CAD build for the part. Positions are in the model's coordinates, mm. Face numbers are marked on the shaded views. A direction names the side the tool comes from. Round coordinates to 2 decimals unless told otherwise and drop trailing zeros. Order: outer loops, then holes, each group sorted by start corner. A loop starts at its lowest first (then second) coordinate and runs counter-clockwise, first axis right, second up. Notation, with made-up numbers: M 33.5,-13 L 64.5,-13 A24 cw 64.5,1 Z; hole C 28.25,55 d4. An arc over 180 degrees is marked long. Answer as a JSON object with one key per item and string values.
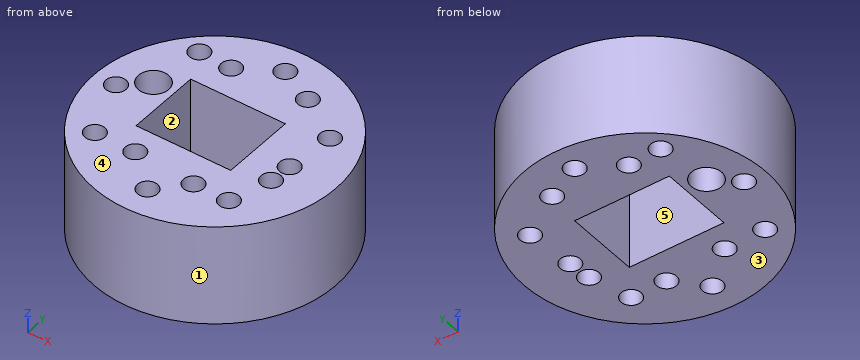
```python
from build123d import *

# Parameters (mm, degrees)
F0_R      = 30
F1_DEPTH  = 25
F2_W      = 23.500042
F2_H      = 18.234876
F3_DEPTH  = 15
F4_DEPTH  = 25
F5_R      = 2.5
F5_R_2    = 3.773073
F6_DEPTH  = 25
F7_R      = 2.5
F8_DEPTH  = 25
F9_R      = 2.5
F10_DEPTH = 25
F11_R     = 2.5
F12_DEPTH = 25


with BuildPart() as f1:
    # F0 (on Top) → F1 (new body)
    with BuildSketch(Plane.XY):
        Circle(F0_R)
    extrude(amount=F1_DEPTH)

    # F2 (on face) → F3 (join)
    with BuildSketch(Plane.XY.offset(25)):
        with Locations((-1.940479, 1.186641)):
            Rectangle(F2_W, F2_H)
    extrude(amount=-F3_DEPTH)

    # F2 (on face) → F4 (cut)
    with BuildSketch(Plane.XY.offset(25)):
        with Locations((-1.940479, 1.186641)):
            Rectangle(F2_W, F2_H)
    extrude(amount=-F4_DEPTH, mode=Mode.SUBTRACT)

    # F5 (on face) → F6 (cut)
    with BuildSketch(Plane.XY.offset(25)):
        with Locations((0, -22.529673)):
            Circle(F5_R)
        with Locations((18.548569, 0)):
            Circle(F5_R)
        with Locations((8.835036, 19.124642)):
            Circle(F5_R)
        with Locations((-19.018844, -14.531934)):
            Circle(F5_R)
        with Locations((-19.018844, 5.049379)):
            Circle(F5_R_2)
    extrude(amount=-F6_DEPTH, mode=Mode.SUBTRACT)

    # F7 (on face) → F8 (cut)
    with BuildSketch(Plane.XY.offset(25)):
        with Locations((-9.274186, 17.875323)):
            Circle(F7_R)
        with Locations((0, 23.479404)):
            Circle(F7_R)
        with Locations((15.148347, -15.728295)):
            Circle(F7_R)
    extrude(amount=-F8_DEPTH, mode=Mode.SUBTRACT)

    # F9 (on face) → F10 (cut)
    with BuildSketch(Plane.XY.offset(25)):
        with Locations((-8.938282, -14.577557)):
            Circle(F9_R)
        with Locations((19.652629, 11.967526)):
            Circle(F9_R)
        with Locations((6.387524, -15.767302)):
            Circle(F9_R)
        with Locations((-24.581272, 0)):
            Circle(F9_R)
        with Locations((-17.395867, 18.182352)):
            Circle(F9_R)
    extrude(amount=-F10_DEPTH, mode=Mode.SUBTRACT)

    # F11 (on face) → F12 (cut)
    with BuildSketch(Plane.XY.offset(25)):
        with Locations((18.113662, -5.651171)):
            Circle(F11_R)
    extrude(amount=-F12_DEPTH, mode=Mode.SUBTRACT)


solid = f1.part
```
Item 1: Drop flat-ended pins along their axis: pin 1 Ø7 at (x, z) = (0.5, 17.5) entering from -Y; pin 2 Ø5.5 at (y, z) = (3.5, 14.5) entering from -X; pin 3 Ø3 at (y, z) = (-17, 15.5) entering from +X. Give the stop position or say it passes through.
Worked answers:
{"pin 1": "stops at y = -30", "pin 2": "stops at x = -29.99", "pin 3": "stops at x = 25.69"}
Item 2: 3-axis set-ups, long thin cutter, end or side, ignore diameter. For the marked faces 4 and 5: which of +Z, -Z, +X, -X, +Y, -Y reach the whole face in a straight line?
Worked answers:
{"face 4": "+Z, +X, -X, +Y, -Y", "face 5": "+Z, -Z"}
Item 3: Saw through at A-A on x = 0. List the corners of the cut face in (y, z), and give its area (3 significant figures).
Worked answers:
{"outline": "M -30,0 L -25.03,0 L -25.03,25 L -30,25 Z; M -20.03,0 L -7.93,0 L -7.93,25 L -20.03,25 Z; M 10.3,0 L 20.98,0 L 20.98,25 L 10.3,25 Z; M 25.98,0 L 30,0 L 30,25 L 25.98,25 Z", "area": "794 mm2"}
Item 4: Saw through at C-C on x = 14. List the corners of the cut face in (y, z).
Worked answers:
{"outline": "M -26.53,0 L -17.95,0 L -17.95,25 L -26.53,25 Z; M -13.51,0 L 26.53,0 L 26.53,25 L -13.51,25 Z"}
Item 5: Saw through at B-B on y = 0. List the corners of the cut face in (x, z), and give its area (4 significant figures).
Worked answers:
{"outline": "M -30,0 L -27.08,0 L -27.08,25 L -30,25 Z; M -22.08,0 L -13.69,0 L -13.69,25 L -22.08,25 Z; M 9.81,0 L 16.05,0 L 16.05,25 L 9.81,25 Z; M 21.05,0 L 30,0 L 30,25 L 21.05,25 Z", "area": "662.5 mm2"}
Item 6: Wall check: line 1 along X through (y, z) = (3, 21.25); line 2 along X through (y, z) = (8, 16); line 3 along Y through (x, z) = (-9, 23.75). Give the ranges that are in metal, low to high. Write a range as [from, to].
Worked answers:
{"line 1": "x = [-29.85, -22.19], [-15.85, -13.69], [9.81, 29.85]", "line 2": "x = [-28.91, -21.37], [-16.67, -13.69], [9.81, 28.91]", "line 3": "y = [-28.62, -17.08], [-12.08, -7.93], [10.3, 15.39], [20.36, 28.62]"}
Item 7: Saw through at D-D on y = -24. List the corners of the cut face in (x, z), and give its area (3 significant figures).
Worked answers:
{"outline": "M -18,0 L -2.02,0 L -2.02,25 L -18,25 Z; M 2.02,0 L 18,0 L 18,25 L 2.02,25 Z", "area": "799 mm2"}
Item 8: Two-plate mould, pull along Y, no slides. Class the marked faces 1, 2 and 3: released by +Y, released by -Y, zero draft, split by the parting line, or undercut.
Worked answers:
{"face 1": "split by the parting line", "face 2": "undercut", "face 3": "zero draft"}
